For this review, take the finished solid that the model builds, in its own axes (mm). A direction names the side the tool comes from. Give positions to 0.01 mm unless a question says otherwise; leave off trailing zeros. Write each loop counter-clockwise with the first axis right and the second up, starting at its lowest first coordinate (ties: lowest second). Pieces come first, ordered by that corner, then holes.
1) Machinability: for faces 1 (the face through (17.45, 4.51, 16.55)), 2 (the face through (8.199, 3.479, 31.067)), 3 (the face through (-0.2, -1.5, 4.3)), 4 (the face through (-16.42, 2.76, 26.11)), which of the approach directions +Z, -Z, +X, -X, +Y, -Y give a long, thin tool a straight path to every point of the face, cutting with its end or side? Answer none if there is none.
2) We need section D-D on z = -7.5. Give the boundary of the cut face in (x, y), and give its area (3 significant figures).
3) For P1, Ø4, axis at x = 15.5, z = 26.95, coming from the -Y side; P2, Ø8, axis at x = 1, z = 6, coming from the +Y side; P3, Ø2.5, axis at x = -15, z = 27, coming from the +Y side, all flat-tipped, find the tip position at first contact; note any pin that passes through.
4) We need section B-B on y = -5.5. Give the boundary of the cut face in (x, z), and give its area (3 significant figures).
5) We need section A-A on y = -3. Give the boundary of the cut face in (x, z), and give its area (3 significant figures).
6) Draft analysis for pull direction X (two halves, no side actions). For faces 5 (the face through (20, 1, 30)), 6 (the face through (-13.53, -2.56, 1.06)), state which applies: pulls with the +X half, pulls with the -X half, needs draft (parallel to the pull), parting line crosses it, or undercut.
7) Wall thickness on line 1 along Z through (x, y) = (0, -4); line 2 along Z through (x, y) = (15.5, 3); line 3 along Z through (x, y) = (1, -8.75): over which ranges is each line inside the solid? List them lowest first.
from build123d import *

# Parameters (mm, degrees)
BOSS_EXTRUDE1_DEPTH = 5
CUT_EXTRUDE6_DEPTH  = 2
CUT_EXTRUDE7_DEPTH  = 2
SKETCH12_R          = 16.732442385
BOSS_EXTRUDE3_DEPTH = 8.6
SKETCH13_R          = 12.1
SKETCH13_R_2        = 10.4
BOSS_EXTRUDE4_DEPTH = 10
SKETCH14_R          = 6
BOSS_EXTRUDE5_DEPTH = 10
CUT_EXTRUDE10_DEPTH = 1
SKETCH7_R           = 1.25
CUT_EXTRUDE11_DEPTH = 19.6
SKETCH8_R           = 2.5
CUT_EXTRUDE12_DEPTH = 1.5
SKETCH3_R           = 15
CUT_EXTRUDE14_DEPTH = 6.5
CUT_EXTRUDE15_DEPTH = 6.5
SKETCH15_R          = 1.25
CUT_EXTRUDE16_DEPTH = 6.5
FILLET2_R           = 1
SKETCH20_R          = 12.503929781
SKETCH20_R_2        = 11.15
CUT_EXTRUDE17_DEPTH = 1
SKETCH21_R          = 4
CUT_EXTRUDE19_DEPTH = 8.8
FILLET10_R          = 1
CUT_EXTRUDE21_DEPTH = 9.6


with BuildPart() as part:
    # Sketch1 → Boss-Extrude1 (new body)
    with BuildSketch(Plane(origin=(0, 0, 0), x_dir=(1, 0, 0), z_dir=(0, 1, 0))):
        with BuildLine():
            Line((-22, -23.004932369), (-22, -33.004932369))
            Line((-22, -33.004932369), (-13.5, -33.004932369))
            Line((-13.5, -33.004932369), (-8.890227771, -30.004932369))
            Line((-8.890227771, -30.004932369), (-7.526591408, -32.100283382))
            ThreePointArc((-7.526591408, -32.100283382), (-3.847417482, -30.904492858), (0, -30.5))
            Line((0, -30.5), (0, 12.5))
            ThreePointArc((0, 12.5), (-7.116131574, 10.276705281), (-11.700861907, 4.397707428))
            Line((-11.700861907, 4.397707428), (-22, -23.004932369))
        make_face()
        with BuildLine():
            ThreePointArc((11.700861907, 4.397707428), (7.116131574, 10.276705281), (0, 12.5))
            Line((0, 12.5), (0, -30.5))
            ThreePointArc((0, -30.5), (3.847417482, -30.904492858), (7.526591408, -32.100283382))
            Line((7.526591408, -32.100283382), (8.890227771, -30.004932369))
            Line((8.890227771, -30.004932369), (13.5, -33.004932369))
            Line((13.5, -33.004932369), (22, -33.004932369))
            Line((22, -33.004932369), (22, -23.004932369))
            Line((22, -23.004932369), (11.700861907, 4.397707428))
        make_face()
    extrude(amount=BOSS_EXTRUDE1_DEPTH)

    # Sketch9 → Cut-Extrude6 (cut)
    with BuildSketch(Plane.XZ):
        with BuildLine():
            Line((20, 33.004932369), (20, 27.004932369))
            ThreePointArc((20, 27.004932369), (0, 18), (-20, 27.004932369))
            Line((-20, 27.004932369), (-20, 33.004932369))
            Line((-20, 33.004932369), (20, 33.004932369))
        make_face()
    extrude(amount=-CUT_EXTRUDE6_DEPTH, mode=Mode.SUBTRACT)

    # Sketch11 → Cut-Extrude7 (cut)
    with BuildSketch(Plane.XZ):
        with BuildLine():
            Line((-20, 23.004932369), (-10.073125454, -3.40723582))
            ThreePointArc((-10.073125454, -3.40723582), (0, -10.633772254), (10.073125454, -3.40723582))
            Line((10.073125454, -3.40723582), (20, 23.004932369))
            Line((20, 23.004932369), (20, 25.529642354))
            ThreePointArc((20, 25.529642354), (0, 17.000016389), (-20, 25.529642354))
            Line((-20, 25.529642354), (-20, 23.004932369))
        make_face()
    extrude(amount=-CUT_EXTRUDE7_DEPTH, mode=Mode.SUBTRACT)

    # Sketch12 → Boss-Extrude3 (add)
    with BuildSketch(Plane.XZ.offset(-5)):
        Circle(SKETCH12_R)
    extrude(amount=BOSS_EXTRUDE3_DEPTH)

    # Sketch13 → Boss-Extrude4 (add)
    with BuildSketch(Plane.XZ.offset(3.6)):
        Circle(SKETCH13_R)
        Circle(SKETCH13_R_2, mode=Mode.SUBTRACT)
    extrude(amount=BOSS_EXTRUDE4_DEPTH)

    # Sketch14 → Boss-Extrude5 (add)
    with BuildSketch(Plane.XZ.offset(3.6)):
        Circle(SKETCH14_R)
    extrude(amount=BOSS_EXTRUDE5_DEPTH)

    # Sketch6 → Cut-Extrude10 (cut)
    with BuildSketch(Plane(origin=(0, 5, 0), x_dir=(1, 0, 0), z_dir=(0, 1, 0))):
        with BuildLine():
            Line((-1.251136393, -17.022628361), (-1.251136393, -26.022628361))
            ThreePointArc((-1.251136393, -26.022628361), (-8.141618616, -27.494920638), (-14.251136393, -31.004932369))
            Line((-14.251136393, -31.004932369), (-20.251136393, -31.004932369))
            Line((-20.251136393, -31.004932369), (-20.251136393, -24.004932369))
            Line((-20.251136393, -24.004932369), (-14.570404486, -8.89036173))
            ThreePointArc((-14.570404486, -8.89036173), (-8.894589877, -14.567823774), (-1.251136393, -17.022628361))
        make_face()
        with BuildLine():
            Line((20.251136393, -24.004932369), (14.570404486, -8.89036173))
            ThreePointArc((14.570404486, -8.89036173), (8.894589877, -14.567823774), (1.251136393, -17.022628361))
            Line((1.251136393, -17.022628361), (1.251136393, -26.022628361))
            ThreePointArc((1.251136393, -26.022628361), (8.141618616, -27.494920638), (14.251136393, -31.004932369))
            Line((14.251136393, -31.004932369), (20.251136393, -31.004932369))
            Line((20.251136393, -31.004932369), (20.251136393, -24.004932369))
        make_face()
    extrude(amount=-CUT_EXTRUDE10_DEPTH, mode=Mode.SUBTRACT)

    # Sketch7 → Cut-Extrude11 (cut, through all)
    with BuildSketch(Plane(origin=(0, 5, 0), x_dir=(1, 0, 0), z_dir=(0, 1, 0))):
        with Locations((-15.5, -26.954932369)):
            Circle(SKETCH7_R)
        with Locations((15.5, -26.954932369)):
            Circle(SKETCH7_R)
    extrude(amount=-CUT_EXTRUDE11_DEPTH, mode=Mode.SUBTRACT)

    # Sketch8 → Cut-Extrude12 (cut)
    with BuildSketch(Plane(origin=(0, 5, 0), x_dir=(1, 0, 0), z_dir=(0, 1, 0))):
        with Locations((-15.5, -26.954932369)):
            Circle(SKETCH8_R)
        with Locations((15.5, -26.954932369)):
            Circle(SKETCH8_R)
    extrude(amount=-CUT_EXTRUDE12_DEPTH, mode=Mode.SUBTRACT)

    # Sketch3 → Cut-Extrude14 (cut)
    with BuildSketch(Plane(origin=(0, 5, 0), x_dir=(1, 0, 0), z_dir=(0, 1, 0))):
        Circle(SKETCH3_R)
    extrude(amount=-CUT_EXTRUDE14_DEPTH, mode=Mode.SUBTRACT)

    # Sketch19 → Cut-Extrude15 (cut)
    with BuildSketch(Plane(origin=(0, 5, 0), x_dir=(1, 0, 0), z_dir=(0, 1, 0))):
        with BuildLine():
            Line((-15.614173224, -6.014334769), (15.614173224, -6.014334769))
            ThreePointArc((15.614173224, -6.014334769), (0, 16.732442385), (-15.614173224, -6.014334769))
        make_face()
    extrude(amount=-CUT_EXTRUDE15_DEPTH, mode=Mode.SUBTRACT)

    # Sketch15 → Cut-Extrude16 (cut)
    with BuildSketch(Plane.XZ.offset(13.6)):
        Circle(SKETCH15_R)
    extrude(amount=-CUT_EXTRUDE16_DEPTH, mode=Mode.SUBTRACT)

    # Fillet2
    fillet2_edges = [part.edges().sort_by_distance(p)[0] for p in [
        (-6, -13.6, 0),
    ]]
    fillet(fillet2_edges, radius=FILLET2_R)

    # Sketch20 → Cut-Extrude17 (cut)
    with BuildSketch(Plane.XZ.offset(13.6)):
        Circle(SKETCH20_R)
        Circle(SKETCH20_R_2, mode=Mode.SUBTRACT)
    extrude(amount=-CUT_EXTRUDE17_DEPTH, mode=Mode.SUBTRACT)

    # Sketch21 → Cut-Extrude19 (cut)
    with BuildSketch(Plane(origin=(0, -1.5, 0), x_dir=(1, 0, 0), z_dir=(0, 1, 0))):
        Circle(SKETCH21_R)
    extrude(amount=-CUT_EXTRUDE19_DEPTH, mode=Mode.SUBTRACT)

    # Fillet10
    fillet10_edges = [part.edges().sort_by_distance(p)[0] for p in [
        (13.741461978, 1.75, 6.014334769),
        (-13.741461978, 1.75, 6.014334769),
    ]]
    fillet(fillet10_edges, radius=FILLET10_R)

    # Sketch22 → Cut-Extrude21 (cut, through all)
    with BuildSketch(Plane.XZ.offset(3.6)):
        with BuildLine():
            Line((15.614173224, 6.014334769), (11.615625162, -3.389284894))
            ThreePointArc((11.615625162, -3.389284894), (0.193858429, -12.098446963), (-11.501074122, -3.759693345))
            Line((-11.501074122, -3.759693345), (-15.614173224, 6.014334769))
            ThreePointArc((-15.614173224, 6.014334769), (0, -16.732442385), (15.614173224, 6.014334769))
        make_face()
    extrude(amount=-CUT_EXTRUDE21_DEPTH, mode=Mode.SUBTRACT)


solid = part.part
Results list:
1. face 1: +Y
1. face 2: +Z, +Y, -Y
1. face 3: -Z, +Y
1. face 4: +Y, -Y
2. outline: (-9.5, -12.6) - (-8.25, -12.6) - (-8.25, -13.6) - (-7.2, -13.6) - (-7.2, -3.6) - (7.2, -3.6) - (7.2, -13.6) - (8.25, -13.6) - (8.25, -12.6) - (9.5, -12.6) - (9.5, -1.5) - (-9.5, -1.5) - close
2. area: 83.2 mm2
3. P1: stops at y = 2
3. P2: stops at y = -1.5
3. P3: stops at y = 3.5
4. outline: circle Ø24.2 at (0, 0); circle Ø12 at (0, 0); hole circle Ø20.8 at (0, 0); hole circle Ø8 at (0, 0)
4. area: 183 mm2
5. outline: (-15.61, 6.01) - (-11.5, -3.76) arc R12.1 ccw to (11.62, -3.39) - (15.61, 6.01) arc R16.73 ccw to start; hole circle Ø8 at (0, 0)
5. area: 598 mm2
6. face 5: undercut
6. face 6: pulls with the -X half
7. line 1: z = -12.1 to -10.4, -6 to -4, 4 to 6, 10.4 to 12.1
7. line 2: z = 6.01 to 25.7, 28.2 to 33
7. line 3: z = -12.06 to -10.35, -5.92 to -3.87, 3.87 to 5.92, 10.35 to 12.06
